Design review of the part built by this model. Coordinates are the model's own, in mm. Face numbers are marked on the shaded views. A direction names the side the tool comes from. Round coordinates to 2 decimals unless told otherwise and drop trailing zeros. Order: outer loops, then holes, each group sorted by start corner. A loop starts at its lowest first (then second) coordinate and runs counter-clockwise, first axis right, second up.
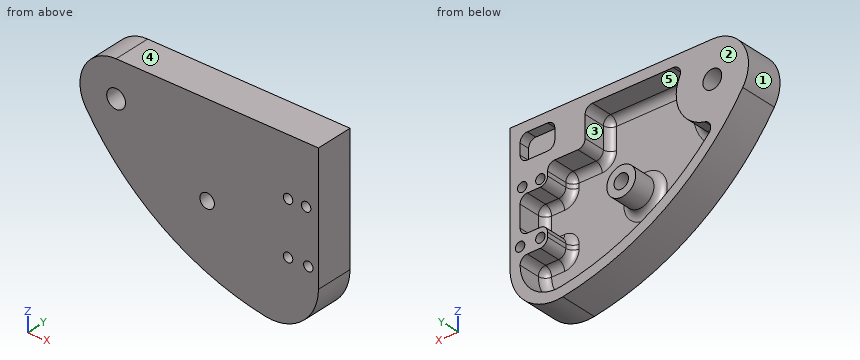
from build123d import *

# Parameters (mm, degrees)
SKETCH1_R             = 3.25
SKETCH1_R_2           = 6.5
BOSS_EXTRUDE1_DEPTH   = 26
SKETCH1_R_3           = 10
SKETCH1_R_4           = 5
BOSS_EXTRUDE1_2_DEPTH = 26
BOSS_EXTRUDE2_DEPTH   = 19
SKETCH1_4_R           = 10
BOSS_EXTRUDE3_DEPTH   = 6
FILLET1_R             = 5


with BuildPart() as part:
    # Sketch1 → Boss-Extrude1 (new body)
    with BuildSketch(Plane(origin=(0, 0, 0), x_dir=(1, 0, 0), z_dir=(0, 1, 0))):
        with BuildLine():
            ThreePointArc((77, 24.5), (65.94372137, 48.579709215), (40.47512467, 55.888900356))
            ThreePointArc((40.47512467, 55.888900356), (-30.523492454, 28.874858685), (-84.055690971, -25.021948297))
            ThreePointArc((-84.055690971, -25.021948297), (-84.931156976, -50.501014695), (-63, -63.5))
            Line((-63, -63.5), (77, -63.5))
            Line((77, -63.5), (77, 24.5))
        make_face()
        with Locations(Location((70, 13, 0), (0, 0, 90))):
            Circle(SKETCH1_R, mode=Mode.SUBTRACT)
        with Locations(Location((56, 13, 0), (0, 0, 90))):
            Circle(SKETCH1_R, mode=Mode.SUBTRACT)
        with Locations(Location((-63, -38.5, 0), (0, 0, 90))):
            Circle(SKETCH1_R_2, mode=Mode.SUBTRACT)
        with Locations(Location((56, -23.5, 0), (0, 0, 90))):
            Circle(SKETCH1_R, mode=Mode.SUBTRACT)
        with Locations(Location((68.5, -23.5, 0), (0, 0, 90))):
            Circle(SKETCH1_R, mode=Mode.SUBTRACT)
        with BuildLine():
            ThreePointArc((-60.54304515, -5.778152172), (-61.597455339, -10.680700417), (-57.867558599, -14.032510442))
            ThreePointArc((-57.867558599, -14.032510442), (-40.575652719, -27.447912005), (-40.469156942, -49.333333333))
            ThreePointArc((-40.469156942, -49.333333333), (-40.195796697, -54.161453237), (-35.962988331, -56.5))
            Line((-35.962988331, -56.5), (20, -56.5))
            ThreePointArc((20, -56.5), (23.535533906, -55.035533906), (25, -51.5))
            Line((25, -51.5), (25, -36.5))
            ThreePointArc((25, -36.5), (26.464466094, -32.964466094), (30, -31.5))
            Line((30, -31.5), (46, -31.5))
            ThreePointArc((46, -31.5), (49.535533906, -30.035533906), (51, -26.5))
            Line((51, -26.5), (51, -23.5))
            ThreePointArc((51, -23.5), (52.464466094, -19.964466094), (56, -18.5))
            Line((56, -18.5), (65, -18.5))
            ThreePointArc((65, -18.5), (68.535533906, -17.035533906), (70, -13.5))
            Line((70, -13.5), (70, 1.5))
            ThreePointArc((70, 1.5), (68.535533906, 5.035533906), (65, 6.5))
            Line((65, 6.5), (56, 6.5))
            ThreePointArc((56, 6.5), (52.464466094, 7.964466094), (51, 11.5))
            Line((51, 11.5), (51, 14.5))
            ThreePointArc((51, 14.5), (52.464466094, 18.035533906), (56, 19.5))
            Line((56, 19.5), (65, 19.5))
            ThreePointArc((65, 19.5), (68.535533906, 20.964466094), (70, 24.5))
            ThreePointArc((70, 24.5), (61.381326107, 43.270796947), (41.527853089, 48.968512876))
            ThreePointArc((41.527853089, 48.968512876), (-14.225405457, 30.391169029), (-60.54304515, -5.778152172))
        make_face(mode=Mode.SUBTRACT)
        with BuildLine():
            Line((46, -51.5), (46, -44))
            ThreePointArc((46, -44), (47.464466094, -40.464466094), (51, -39))
            Line((51, -39), (65, -39))
            ThreePointArc((65, -39), (68.535533906, -40.464466094), (70, -44))
            Line((70, -44), (70, -51.5))
            ThreePointArc((70, -51.5), (68.535533906, -55.035533906), (65, -56.5))
            Line((65, -56.5), (51, -56.5))
            ThreePointArc((51, -56.5), (47.464466094, -55.035533906), (46, -51.5))
        make_face(mode=Mode.SUBTRACT)
    extrude(amount=BOSS_EXTRUDE1_DEPTH)

    # Sketch1_3 → Boss-Extrude2 (add)
    with BuildSketch(Plane(origin=(0, 0, 0), x_dir=(1, 0, 0), z_dir=(0, 1, 0))):
        with BuildLine():
            ThreePointArc((46, -44), (47.464466094, -40.464466094), (51, -39))
            Line((51, -39), (65, -39))
            ThreePointArc((65, -39), (68.535533906, -40.464466094), (70, -44))
            Line((70, -44), (70, -51.5))
            ThreePointArc((70, -51.5), (68.535533906, -55.035533906), (65, -56.5))
            Line((65, -56.5), (51, -56.5))
            ThreePointArc((51, -56.5), (47.464466094, -55.035533906), (46, -51.5))
            Line((46, -51.5), (46, -44))
        make_face()
    extrude(amount=BOSS_EXTRUDE2_DEPTH)



with BuildPart() as body_2:
    # Sketch1 → Boss-Extrude1 2 (new body)
    with BuildSketch(Plane(origin=(0, 0, 0), x_dir=(1, 0, 0), z_dir=(0, 1, 0))):
        with Locations(Location((0, 0, 0), (0, 0, 90))):
            Circle(SKETCH1_R_3)
        with Locations(Location((0, 0, 0), (0, 0, 90))):
            Circle(SKETCH1_R_4, mode=Mode.SUBTRACT)
    extrude(amount=BOSS_EXTRUDE1_2_DEPTH)


with BuildPart() as part_1:
    add(part.part)

    add(body_2.part)  # Boss-Extrude3 merges body 2
    # Sketch1_4 → Boss-Extrude3 (add)
    with BuildSketch(Plane(origin=(0, 0, 0), x_dir=(1, 0, 0), z_dir=(0, 1, 0))):
        with BuildLine():
            ThreePointArc((41.527853089, 48.968512876), (-14.225405457, 30.391169029), (-60.54304515, -5.778152172))
            ThreePointArc((-60.54304515, -5.778152172), (-61.597455339, -10.680700417), (-57.867558599, -14.032510442))
            ThreePointArc((-57.867558599, -14.032510442), (-40.575652719, -27.447912005), (-40.469156942, -49.333333333))
            ThreePointArc((-40.469156942, -49.333333333), (-40.195796697, -54.161453237), (-35.962988331, -56.5))
            Line((-35.962988331, -56.5), (20, -56.5))
            ThreePointArc((20, -56.5), (23.535533906, -55.035533906), (25, -51.5))
            Line((25, -51.5), (25, -36.5))
            ThreePointArc((25, -36.5), (26.464466094, -32.964466094), (30, -31.5))
            Line((30, -31.5), (46, -31.5))
            ThreePointArc((46, -31.5), (49.535533906, -30.035533906), (51, -26.5))
            Line((51, -26.5), (51, -23.5))
            ThreePointArc((51, -23.5), (52.464466094, -19.964466094), (56, -18.5))
            Line((56, -18.5), (65, -18.5))
            ThreePointArc((65, -18.5), (68.535533906, -17.035533906), (70, -13.5))
            Line((70, -13.5), (70, 1.5))
            ThreePointArc((70, 1.5), (68.535533906, 5.035533906), (65, 6.5))
            Line((65, 6.5), (56, 6.5))
            ThreePointArc((56, 6.5), (52.464466094, 7.964466094), (51, 11.5))
            Line((51, 11.5), (51, 14.5))
            ThreePointArc((51, 14.5), (52.464466094, 18.035533906), (56, 19.5))
            Line((56, 19.5), (65, 19.5))
            ThreePointArc((65, 19.5), (68.535533906, 20.964466094), (70, 24.5))
            ThreePointArc((70, 24.5), (61.381326107, 43.270796947), (41.527853089, 48.968512876))
        make_face()
        with Locations(Location((0, 0, 0), (0, 0, 90))):
            Circle(SKETCH1_4_R, mode=Mode.SUBTRACT)
    extrude(amount=BOSS_EXTRUDE3_DEPTH)

    # Fillet1
    fillet1_edges = [part_1.edges().sort_by_distance(p)[0] for p in [
        (-40.575652719, 6, 27.447912005),
        (-40.195796697, 6, 54.161453237),
        (0, 6, 10),
        (-14.225405457, 6, -30.391169029),
        (-61.597455339, 6, 10.680700417),
        (-7.981494165, 6, 56.5),
        (23.535533906, 6, 55.035533906),
        (25, 6, 44),
        (26.464466094, 6, 32.964466094),
        (38, 6, 31.5),
        (49.535533906, 6, 30.035533906),
        (51, 6, 25),
        (52.464466094, 6, 19.964466094),
        (60.5, 6, 18.5),
        (68.535533906, 6, 17.035533906),
        (70, 6, 6),
        (68.535533906, 6, -5.035533906),
        (60.5, 6, -6.5),
        (52.464466094, 6, -7.964466094),
        (51, 6, -13),
        (52.464466094, 6, -18.035533906),
        (60.5, 6, -19.5),
        (68.535533906, 6, -20.964466094),
        (61.381326107, 6, -43.270796947),
    ]]
    fillet(fillet1_edges, radius=FILLET1_R)


solid = part_1.part
1) For the marked faces 4 and 5, list the 3-axis set-ups (+Z, -Z, +X, -X, +Y, -Y) from which the entire face can be reached by the end or side of a thin tool; tool diameter is ignored.
Results:
face 4: +Z, +X, -X, +Y, -Y
face 5: +Y
2) The part is to be moulded in two halves that separate along Z. For the marked faces 1, 2 and 3, say which applies: released by +Z, released by -Z, zero draft, split by the parting line, or undercut.
Results:
face 1: split by the parting line
face 2: zero draft
face 3: undercut
3) Clearance check with flat-ended pins moving along their axes: P1, Ø7, axis at x = 62.5, y = 18.5, coming from the -Z side; P2, Ø14, axis at x = 60.5, z = 48.5, coming from the +Y side; P3, Ø9, axis at x = 0, z = 0, coming from the +Y side; P4, Ø8, axis at y = 22.5, z = -8.5, coming from the -X side. State where each tip first meets the part, or that it passes through.
Results:
P1: stops at z = -53.12
P2: stops at y = 19
P3: passes through
P4: stops at x = -60.45
4) Take a section at A-A on z = 54.5. Give the boundary of the cut face in (x, y), plus the area to 3 significant figures.
Results:
outline: (-82.21, 0) - (77, 0) - (77, 26) - (69, 26) - (69, 19) - (47, 19) - (47, 26) - (24, 26) - (24, 11) arc R4 cw to (20, 7) - (-35.96, 7) arc R4 cw to (-39.96, 11) - (-39.96, 26) - (-82.21, 26) - close
area: 2,780 mm2
5) To check wall thickness, follow line 1 along Z through (x, y) = (61, 8); line 2 along X through (y, z) = (22.25, 3); line 3 along X through (y, z) = (12.25, -5.5). State the ranges of each line that lie inside material, in increasing order.
Results:
line 1: z = -52.07 to -42.28, -20.5 to -5.5, 17.5 to 63.5
line 2: x = -67.45 to -57.96, -9.54 to -4, 4 to 9.54, 70 to 77
line 3: x = -59.45 to -49.32, -8.35 to 8.35, 68 to 77
